Could you check a few things on this model? Use its own coordinates, in mm. A direction names the side the tool comes from. Round coordinates to 2 decimals unless told otherwise and drop trailing zeros. Write each loop counter-clockwise with the first axis right and the second up, starting at its lowest first coordinate (ties: lowest second). Pieces come first, ordered by that corner, then holes. Notation, with made-up numbers: (44, 4.25) - (69, 4.25) arc R22 cw to (69, 42.25) - close; hole circle Ø9 at (81.25, 17). An arc over 180 degrees is marked (long way). Put each result on its own line as item: value.
from build123d import *

# Parameters (mm, degrees)
F0_W     = 24
F0_H     = 4
F0_R     = 2
F1_DEPTH = 2.5


with BuildPart() as f1:
    # F0 (on Top) → F1 (new body)
    with BuildSketch(Plane.XY):
        with BuildLine():
            Line((-36.882881, 6.197646), (-51.882881, 6.197646))
            ThreePointArc((-51.882881, 6.197646), (-55.418415, 4.73318), (-56.882881, 1.197646))
            Line((-56.882881, 1.197646), (-56.882881, -26.802354))
            ThreePointArc((-56.882881, -26.802354), (-55.418415, -30.337887), (-51.882881, -31.802354))
            Line((-51.882881, -31.802354), (-8.882881, -31.802354))
            Line((-8.882881, -31.802354), (-8.882881, -27.802354))
            Line((-8.882881, -27.802354), (15.117119, -27.802354))
            Line((15.117119, -27.802354), (15.117119, -31.802354))
            Line((15.117119, -31.802354), (58.117119, -31.802354))
            ThreePointArc((58.117119, -31.802354), (61.652653, -30.337887), (63.117119, -26.802354))
            Line((63.117119, -26.802354), (63.117119, 1.197646))
            ThreePointArc((63.117119, 1.197646), (61.652653, 4.73318), (58.117119, 6.197646))
            Line((58.117119, 6.197646), (43.117119, 6.197646))
            Line((43.117119, 6.197646), (23.117119, 6.197646))
            Line((23.117119, 6.197646), (23.117119, 41.197646))
            ThreePointArc((23.117119, 41.197646), (21.652653, 44.73318), (18.117119, 46.197646))
            Line((18.117119, 46.197646), (-11.882881, 46.197646))
            ThreePointArc((-11.882881, 46.197646), (-15.418415, 44.73318), (-16.882881, 41.197646))
            Line((-16.882881, 41.197646), (-16.882881, 6.197646))
            Line((-16.882881, 6.197646), (-36.882881, 6.197646))
        make_face()
        with Locations((3.117119, 4.197646)):
            Rectangle(F0_W, F0_H, mode=Mode.SUBTRACT)
        with Locations((-11.882881, 11.197646)):
            Circle(F0_R, mode=Mode.SUBTRACT)
        with Locations((-11.882881, 41.197646)):
            Circle(F0_R, mode=Mode.SUBTRACT)
        with Locations((18.117119, 11.197646)):
            Circle(F0_R, mode=Mode.SUBTRACT)
        with Locations((18.117119, 41.197646)):
            Circle(F0_R, mode=Mode.SUBTRACT)
        with BuildLine():
            Line((-36.882881, 41.197646), (-36.882881, 6.197646))
            Line((-36.882881, 6.197646), (-16.882881, 6.197646))
            Line((-16.882881, 6.197646), (-16.882881, 41.197646))
            ThreePointArc((-16.882881, 41.197646), (-15.418415, 44.73318), (-11.882881, 46.197646))
            Line((-11.882881, 46.197646), (-16.882881, 46.197646))
            Line((-16.882881, 46.197646), (-31.882881, 46.197646))
            ThreePointArc((-31.882881, 46.197646), (-35.418415, 44.73318), (-36.882881, 41.197646))
        make_face()
        with BuildLine():
            Line((23.117119, 46.197646), (18.117119, 46.197646))
            ThreePointArc((18.117119, 46.197646), (21.652653, 44.73318), (23.117119, 41.197646))
            Line((23.117119, 41.197646), (23.117119, 6.197646))
            Line((23.117119, 6.197646), (43.117119, 6.197646))
            Line((43.117119, 6.197646), (43.117119, 41.197646))
            ThreePointArc((43.117119, 41.197646), (41.652653, 44.73318), (38.117119, 46.197646))
            Line((38.117119, 46.197646), (23.117119, 46.197646))
        make_face()
    extrude(amount=F1_DEPTH)


solid = f1.part
(1) Imagine slicing it at C-C, the plane x = -47. List the corners of the cut face in (y, z) for me.
Values found:
outline: (-31.8, 0) - (6.2, 0) - (6.2, 2.5) - (-31.8, 2.5) - close
(2) I'm going to push flat-ended pins straight in: pin 1 (4.5 mm diameter, centred on x = -11.88, y = 41.2, fed in from -Z); pin 2 (1.2 mm diameter, centred on y = 4, z = 1, fed in from -X); pin 3 (1.2 mm diameter, centred on y = 16, z = 1, fed in from -X); pin 4 (1.2 mm diameter, centred on y = -30, z = 1, fed in from +X). Where does each tip first touch, or does it pass through?
Values found:
pin 1: stops at z = 0
pin 2: stops at x = -56.37
pin 3: stops at x = -36.88
pin 4: stops at x = 62.39
(3) Imagine slicing it at B-B, the plane z = 0.9. List the corners of the cut face in (x, y) for me.
Values found:
outline: (-56.88, -26.8) arc R5 ccw to (-51.88, -31.8) - (-8.88, -31.8) - (-8.88, -27.8) - (15.12, -27.8) - (15.12, -31.8) - (58.12, -31.8) arc R5 ccw to (63.12, -26.8) - (63.12, 1.2) arc R5 ccw to (58.12, 6.2) - (43.12, 6.2) - (43.12, 41.2) arc R5 ccw to (38.12, 46.2) - (-31.88, 46.2) arc R5 ccw to (-36.88, 41.2) - (-36.88, 6.2) - (-51.88, 6.2) arc R5 ccw to (-56.88, 1.2) - close; hole circle Ø4 at (-11.88, 11.2); hole circle Ø4 at (-11.88, 41.2); hole (-8.88, 2.2) - (15.12, 2.2) - (15.12, 6.2) - (-8.88, 6.2) - close; hole circle Ø4 at (18.12, 11.2); hole circle Ø4 at (18.12, 41.2)
(4) Imagine slicing it at D-D, the plane y = 21. List the corners of the cut face in (x, z) for me, then the cut area to 3 significant figures.
Values found:
outline: (-36.88, 0) - (43.12, 0) - (43.12, 2.5) - (-36.88, 2.5) - close
area: 200 mm^2
(5) Please list where these lines run through material, in increasing order: probe 1 along X at (y, z) = (11.5, 0.95); probe 2 along Y at (x, z) = (-7, 2.15); probe 3 along Y at (x, z) = (-39, 2.4). Write a range as from..to.
Values found:
probe 1: x = -36.88..-13.86, -9.91..16.14, 20.09..43.12
probe 2: y = -27.8..2.2, 6.2..46.2
probe 3: y = -31.8..6.2
(6) For faces 4 (the face through (-35.38, 44.77, 1.23)), 5 (the face through (3, -27.802, 1)), 6 (the face through (3, 6.198, 1)), 7 (the face through (43.117, 23, 1)), which set-ups out of +Z, -Z, +X, -X, +Y, -Y let a thin tool reach every point of the face, with its end or its side?
Values found:
face 4: +Z, -Z, -X, +Y
face 5: +Z, -Z, -Y
face 6: +Z, -Z
face 7: +Z, -Z, +X, +Y
(7) If we mould it in two halves opening along X, with no side actions, what happens to faces 1 (the face through (-55.38, 4.77, 1.23)), 2 (the face through (-44, 6.198, 1)), 3 (the face through (-8.883, 4, 1))? For each: pulls with the +X half, pulls with the -X half, needs draft (parallel to the pull), parting line crosses it, or undercut.
Values found:
face 1: pulls with the -X half
face 2: needs draft
face 3: undercut
(8) Imagine slicing it at A-A, the plane x = 3. List the corners of the cut face in (y, z) for me.
Values found:
outline: (-27.8, 0) - (2.2, 0) - (2.2, 2.5) - (-27.8, 2.5) - close; (6.2, 0) - (46.2, 0) - (46.2, 2.5) - (6.2, 2.5) - close
